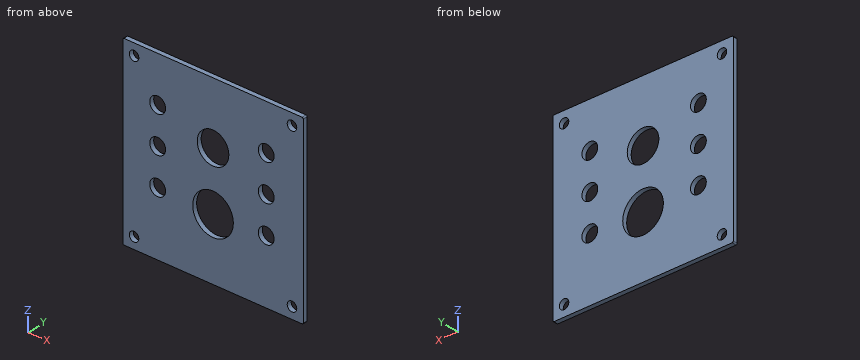
```python
from build123d import *

# Parameters (mm, degrees)
F0_R     = 3.3528
F0_R_2   = 5.5626
F0_R_3   = 14.29385
F0_R_4   = 11.11885
F1_DEPTH = 3.175


with BuildPart() as f1:
    # F0 (on Front) → F1 (new body)
    with BuildSketch(Plane.XZ):
        with BuildLine():
            ThreePointArc((0, 0.7874), (0.230624, 0.230624), (0.7874, 0))
            Line((0.7874, 0), (126.2126, 0))
            ThreePointArc((126.2126, 0), (126.769376, 0.230624), (127, 0.7874))
            Line((127, 0.7874), (127, 126.2126))
            ThreePointArc((127, 126.2126), (126.769376, 126.769376), (126.2126, 127))
            Line((126.2126, 127), (0.7874, 127))
            ThreePointArc((0.7874, 127), (0.230624, 126.769376), (0, 126.2126))
            Line((0, 126.2126), (0, 0.7874))
        make_face()
        with Locations((7.9248, 7.9248)):
            Circle(F0_R, mode=Mode.SUBTRACT)
        with Locations((24.5364, 44.45)):
            Circle(F0_R_2, mode=Mode.SUBTRACT)
        with Locations((119.0752, 7.9248)):
            Circle(F0_R, mode=Mode.SUBTRACT)
        with Locations((63.5, 43.1546)):
            Circle(F0_R_3, mode=Mode.SUBTRACT)
        with Locations((100.9396, 44.45)):
            Circle(F0_R_2, mode=Mode.SUBTRACT)
        with Locations((24.5364, 69.85)):
            Circle(F0_R_2, mode=Mode.SUBTRACT)
        with Locations((24.5364, 95.25)):
            Circle(F0_R_2, mode=Mode.SUBTRACT)
        with Locations((7.9248, 119.0752)):
            Circle(F0_R, mode=Mode.SUBTRACT)
        with Locations((63.5, 83.8454)):
            Circle(F0_R_4, mode=Mode.SUBTRACT)
        with Locations((100.9396, 69.85)):
            Circle(F0_R_2, mode=Mode.SUBTRACT)
        with Locations((100.9396, 95.25)):
            Circle(F0_R_2, mode=Mode.SUBTRACT)
        with Locations((119.0752, 119.0752)):
            Circle(F0_R, mode=Mode.SUBTRACT)
    extrude(amount=F1_DEPTH)


solid = f1.part
```
The listing builds one solid part. Answer for the finished solid, in the listing's coordinates (mm). Give positions to 0.01 mm unless a question says otherwise; leave off trailing zeros. Order: outer loops, then holes, each group sorted by start corner. A loop starts at its lowest first (then second) coordinate and runs counter-clockwise, first axis right, second up. Notation, with made-up numbers: (-3.5, 60) -> (55.5, 60) arc R19 ccw to (55.5, 77) -> close; hole circle Ø1 at (31, 39.5). An arc over 180 degrees is marked (long way). Answer as a JSON object with one key per item and string values. Group by question number.
Item 1: A flat-ended cylindrical pin translates along its axis: pin 1 (6.5 mm diameter, centred on x = 100.94, z = 44.45, fed in from +Y). Find the tip coordinate at first contact, or state that the pin passes through.
Item 2: Consider L1, parallel to Z at x = 63.5, y = -1.7; L2, parallel to X at y = -2.25, z = 69.5; L3, parallel to Z at x = 104.5, y = -1.55. Determine where each line is inside the solid, lowest interval first. Write a range as from..to.
Item 3: The part is cut by section B-B on x = 63.5. Write down the section's boundary in (y, z) (3 decimals).
Item 4: The part is cut by section C-C on y = -0.7. Give the number of separate pieces and of enclosed holes in the cut face, and give its area (3 significant figures).
Item 5: The part is cut by section A-A on z = 69.85. Write down the section's boundary in (x, y) (3 decimals).
Result set:
{
 "1": {"pin 1": "through"},
 "2": {"L1": "0..28.86, 57.45..72.73, 94.96..127", "L2": "0..18.98, 30.09..95.39, 106.49..127", "L3": "0..40.18, 48.72..65.58, 74.12..90.98, 99.52..127"},
 "3": {"outline": "(-3.175, 0) -> (0, 0) -> (0, 28.861) -> (-3.175, 28.861) -> close; (-3.175, 57.448) -> (0, 57.448) -> (0, 72.727) -> (-3.175, 72.727) -> close; (-3.175, 94.964) -> (0, 94.964) -> (0, 127) -> (-3.175, 127) -> close"},
 "4": {"separate pieces": "1", "enclosed holes": "12", "area": "14,400 mm²"},
 "5": {"outline": "(0, -3.175) -> (18.974, -3.175) -> (18.974, 0) -> (0, 0) -> close; (30.099, -3.175) -> (95.377, -3.175) -> (95.377, 0) -> (30.099, 0) -> close; (106.502, -3.175) -> (127, -3.175) -> (127, 0) -> (106.502, 0) -> close"}
}
